Build history of the part. All positions in model axes, mm. A direction names the side the tool comes from. Give positions to 0.01 mm unless a question says otherwise; leave off trailing zeros. Order: outer loops, then holes, each group sorted by start corner. A loop starts at its lowest first (then second) coordinate and runs counter-clockwise, first axis right, second up. Notation, with made-up numbers: M -25.75,64.25 L -19.75,64.25 A16 cw -19.75,81.25 Z; hole C 69.5,74.25 d11. An arc over 180 degrees is marked long. Answer as CSV lines item,"result".
from build123d import *

# Parameters (mm, degrees)
SKETCH_1_W          = 10.5
SKETCH_1_H          = 36
EXTRUDE_1_DEPTH     = 2
SKETCH_2_R          = 1.6
CUT_EXTRUDE_1_DEPTH = 3
SKETCH_3_W          = 9
SKETCH_3_H          = 25
CUT_EXTRUDE_2_DEPTH = 1
SKETCH_6_W          = 0.75
SKETCH_6_H          = 1
CUT_EXTRUDE_3_DEPTH = 0.5
SKETCH_7_W          = 4.3
SKETCH_7_H          = 5.5
CUT_EXTRUDE_4_DEPTH = 0.2


with BuildPart() as part:
    # 草图1 → 凸台-拉伸1 (new body)
    with BuildSketch(Plane(origin=(0, 0, 0), x_dir=(1, 0, 0), z_dir=(0, 1, 0))):
        with Locations((5.25, 18)):
            Rectangle(SKETCH_1_W, SKETCH_1_H)
    extrude(amount=EXTRUDE_1_DEPTH)

    # 草图2 → 切除-拉伸1 (cut, through all)
    with BuildSketch(Plane(origin=(0, 0, 0), x_dir=(-1, 0, 0), z_dir=(0, -1, 0))):
        with Locations((-7.5, 33)):
            Circle(SKETCH_2_R)
        with Locations((-7.5, 3)):
            Circle(SKETCH_2_R)
    extrude(amount=-CUT_EXTRUDE_1_DEPTH, mode=Mode.SUBTRACT)

    # 草图3 → 切除-拉伸2 (cut)
    with BuildSketch(Plane(origin=(0, 0, 0), x_dir=(-1, 0, 0), z_dir=(0, -1, 0))):
        with Locations((-5.25, 18)):
            Rectangle(SKETCH_3_W, SKETCH_3_H)
    extrude(amount=-CUT_EXTRUDE_2_DEPTH, mode=Mode.SUBTRACT)

    # 草图6 → 切除-拉伸3 (cut)
    with BuildSketch(Plane(origin=(0, 0, 0), x_dir=(-1, 0, 0), z_dir=(0, -1, 0))):
        with Locations((-0.375, 17.5)):
            Rectangle(SKETCH_6_W, SKETCH_6_H)
    extrude(amount=-CUT_EXTRUDE_3_DEPTH, mode=Mode.SUBTRACT)

    # 草图7 → 切除-拉伸4 (cut)
    with BuildSketch(Plane(origin=(0, 0, 0), x_dir=(-1, 0, 0), z_dir=(0, -1, 0))):
        with Locations((-3.15, 33.25)):
            Rectangle(SKETCH_7_W, SKETCH_7_H)
    extrude(amount=-CUT_EXTRUDE_4_DEPTH, mode=Mode.SUBTRACT)


solid = part.part
Item 1: Band-saw the part on A-A (z = -3). Give the cut face in (x, y), and give its area (3 significant figures).
Geometry says:
outline,"M 0,0 L 5.9,0 L 5.9,2 L 0,2 Z; M 9.1,0 L 10.5,0 L 10.5,2 L 9.1,2 Z"
area,"14.6 mm2"
Item 2: Band-saw the part on B-B (x = 7.5). Give the cut face in (y, z), and give its area (3 significant figures).
Geometry says:
outline,"M 0,-36 L 2,-36 L 2,-34.6 L 0,-34.6 Z; M 0,-31.4 L 2,-31.4 L 2,-4.6 L 0,-4.6 L 0,-5.5 L 1,-5.5 L 1,-30.5 L 0,-30.5 Z; M 0,-1.4 L 2,-1.4 L 2,0 L 0,0 Z"
area,"34.2 mm2"
Item 3: Band-saw the part on C-C (z = -27.5). Give the cut face in (x, y), and give its area (3 significant figures).
Geometry says:
outline,"M 0,0 L 0.75,0 L 0.75,1 L 9.75,1 L 9.75,0 L 10.5,0 L 10.5,2 L 0,2 Z"
area,"12.0 mm2"
Item 4: 3-axis set-ups, long thin cutter, end or side, ignore diameter. For faces 5 (the flat face through (0.75, 0.7, -17.8)), 6 (the cylindrical face through (8.77, 0.99, -2.03)), 7 (the flat face through (3, 0.2, -33)): which of +Z, -Z, +X, -X, +Y, -Y reach the whole face in a straight line?
Geometry says:
face 5,"-Y"
face 6,"+Y, -Y"
face 7,"-Z, -Y"
Item 5: Pull direction Z, two halves, no side cores. Call faces 1 (the flat face through (5, 1, -36)), 2 (the flat face through (5, 1, -18)), 3 (the cylindrical face through (7.85, 0.99, -31.44)), 4 (the flat face through (0.4, 0, -27.1)): released by +Z, released by -Z, zero draft, split by the parting line, or undercut.
Geometry says:
face 1,"released by -Z"
face 2,"undercut"
face 3,"undercut"
face 4,"zero draft"
Item 6: Probe line 1 along Z through (x, y) = (7.5, 1.3); line 2 along Z through (x, y) = (7.5, 0.95); line 3 along X through (y, z) = (0.95, -33). List the from-to ranges inside material, lowest first. Write a range as from..to.
Geometry says:
line 1,"z = -36..-34.6, -31.4..-4.6, -1.4..0"
line 2,"z = -36..-34.6, -31.4..-30.5, -5.5..-4.6, -1.4..0"
line 3,"x = 0..5.9, 9.1..10.5"
Item 7: Drop a flat-ended pin along its axis: pin 1 (2 mm diameter, centred on x = 4, z = -34, fed in from -Y). Give the stop position or say it passes through.
Geometry says:
pin 1,"stops at y = 0.2"
Item 8: Band-saw the part on D-D (y = 1.7). Give the cut face in (x, z), and give its area (3 significant figures).
Geometry says:
outline,"M 0,-36 L 10.5,-36 L 10.5,0 L 0,0 Z; hole C 7.5,-33 d3.2; hole C 7.5,-3 d3.2"
area,"362 mm2"
